Design review of the part built by this model. Coordinates are the model's own, in mm. Face numbers are marked on the shaded views. A direction names the side the tool comes from. Coordinates: 2 decimals unless noted, no trailing zeros. Write each loop counter-clockwise with the first axis right and the second up, starting at its lowest first coordinate (ties: lowest second). Pieces come first, ordered by that corner, then holes. Notation, with made-up numbers: (12.5, -22) - (68.5, -22) arc R27 cw to (68.5, 6) - close; hole circle Ø1 at (-7, -35). An arc over 180 degrees is marked (long way). One line per item, written item: value.
from build123d import *

# Parameters (mm, degrees)
SKETCH1_W           = 4
SKETCH1_H           = 1
BOSS_EXTRUDE1_DEPTH = 10
SKETCH11_W          = 4
SKETCH11_H          = 1
BOSS_EXTRUDE2_DEPTH = 11
SKETCH12_R          = 1.5
CUT_EXTRUDE1_DEPTH  = 10
SKETCH13_R          = 1.5
CUT_EXTRUDE2_DEPTH  = 10


with BuildPart() as part:
    # Sketch1 → Boss-Extrude1 (new body)
    with BuildSketch(Plane.XY):
        Rectangle(SKETCH1_W, SKETCH1_H)
    extrude(amount=BOSS_EXTRUDE1_DEPTH)

    # Sketch11 → Boss-Extrude2 (add)
    with BuildSketch(Plane(origin=(0, 0.5, 0), x_dir=(1, 0, 0), z_dir=(0, 1, 0))):
        with Locations((0, -0.5)):
            Rectangle(SKETCH11_W, SKETCH11_H)
    extrude(amount=BOSS_EXTRUDE2_DEPTH)

    # Sketch12 → Cut-Extrude1 (cut)
    with BuildSketch(Plane(origin=(0, 0.5, 0), x_dir=(1, 0, 0), z_dir=(0, 1, 0))):
        with Locations(Location((0, -5.6, 0), (0, 0, 180))):
            Circle(SKETCH12_R)
    extrude(amount=-CUT_EXTRUDE1_DEPTH, mode=Mode.SUBTRACT)

    # Sketch13 → Cut-Extrude2 (cut)
    with BuildSketch(Plane.XY.offset(1)):
        with Locations((0, 5.5)):
            Circle(SKETCH13_R)
    extrude(amount=-CUT_EXTRUDE2_DEPTH, mode=Mode.SUBTRACT)


solid = part.part
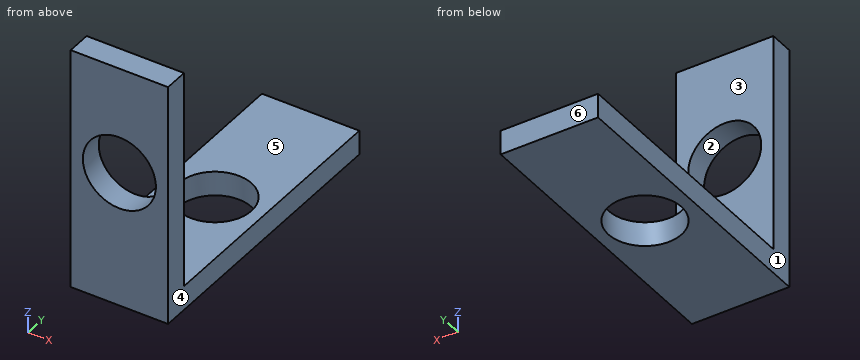
1. Wall thickness on line 1 along Y through (x, z) = (0, 0.6); line 2 along Z through (x, y) = (0, -0.2); line 3 along Z through (x, y) = (-0.55, 2.75): over which ranges is each line inside the solid? List them lowest first.
Answer block:
line 1: y = -0.5 to 4, 7 to 11.5
line 2: z = 0 to 4.1, 7.1 to 10
line 3: z = 0 to 1
2. Consider section B-B, the plane z = 5.6. Write out the cut boundary in (x, y).
Answer block:
outline: (-2, -0.5) - (-1.5, -0.5) - (-1.5, 0.5) - (-2, 0.5) - close; (1.5, -0.5) - (2, -0.5) - (2, 0.5) - (1.5, 0.5) - close
3. Consider section C-C, the plane x = 0. Write out the cut boundary in (y, z), then the cut area to 3 significant figures.
Answer block:
outline: (-0.5, 0) - (4, 0) - (4, 1) - (0.5, 1) - (0.5, 4.1) - (-0.5, 4.1) - close; (-0.5, 7.1) - (0.5, 7.1) - (0.5, 10) - (-0.5, 10) - close; (7, 0) - (11.5, 0) - (11.5, 1) - (7, 1) - close
area: 15.0 mm^2
4. Mouldability with a two-part tool opening along X and no side actions: class the marked faces 1, 2, 3 and 4 as released by +X, released by -X, zero draft, split by the parting line, or undercut.
Answer block:
face 1: released by -X
face 2: undercut
face 3: zero draft
face 4: released by +X
5. For the marked faces 5 and 6, list the 3-axis set-ups (+Z, -Z, +X, -X, +Y, -Y) from which the entire face can be reached by the end or side of a thin tool; tool diameter is ignored.
Answer block:
face 5: +Z, +X, -X, +Y
face 6: +Z, -Z, +X, -X, +Y
6. Consider section D-D, the plane x = 1.7. Write out the cut boundary in (y, z).
Answer block:
outline: (-0.5, 0) - (11.5, 0) - (11.5, 1) - (0.5, 1) - (0.5, 10) - (-0.5, 10) - close
7. Consider section A-A, the plane y = 5.5. Write out the cut boundary in (x, z), then the cut area to 3 significant figures.
Answer block:
outline: (-2, 0) - (-1.5, 0) - (-1.5, 1) - (-2, 1) - close; (1.5, 0) - (2, 0) - (2, 1) - (1.5, 1) - close
area: 1.00 mm^2
